The model under review builds one solid part; all positions refer to its coordinate system, in mm. Face numbers are marked on the shaded views. A direction names the side the tool comes from. Coordinates: 2 decimals unless noted, no trailing zeros. Order: outer loops, then holes, each group sorted by start corner. A loop starts at its lowest first (then second) coordinate and runs counter-clockwise, first axis right, second up. Notation, with made-up numbers: (87.5, -40) -> (125.5, -40) arc R16 ccw to (125.5, -10) -> close; hole circle Ø2 at (-2.75, -34.75). An arc over 180 degrees is marked (long way). Use one line per item in the form item = value.
from build123d import *

# Parameters (mm, degrees)
SKETCH_R           = 15
PAD_DEPTH          = 108
PAD_TAPER          = -10
SKETCH001_R        = 72.5
PAD001_DEPTH       = 14
POCKET_DEPTH       = 571.52662
PAD002_DEPTH       = 2.5
POLARPATTERN_COUNT = 6


with BuildPart() as part:
    # Sketch (on XY_Plane of Origin) → Pad (new body)
    with BuildSketch(Plane.XY):
        Circle(SKETCH_R)
    extrude(amount=-PAD_DEPTH, taper=PAD_TAPER)

    # Sketch001 (on Face3 of Pad) → Pad001 (join)
    with BuildSketch(Plane(origin=(0, 0, -108), x_dir=(1, 0, 0), z_dir=(0, 0, -1))):
        Circle(SKETCH001_R)
    extrude(amount=-PAD001_DEPTH)

    # Sketch002 (on XY_Plane of Origin) → Pocket (cut, through all)
    with BuildSketch(Plane.XY):
        with BuildLine():
            Line((-31.369354, -65.362173), (-22.5, -50))
            Line((-22.5, -50), (22.5, -50))
            Line((22.5, -50), (31.369354, -65.362173))
            ThreePointArc((-31.369354, -65.362173), (0, -72.5), (31.369354, -65.362173))
        make_face()
    pocket = extrude(amount=-POCKET_DEPTH, mode=Mode.SUBTRACT)

    # Mirrored: Pocket across XZ
    add(pocket.mirror(Plane.XZ), mode=Mode.SUBTRACT)

    # Sketch003 (on XZ_Plane of Origin) → Groove (revolve, cut)
    with BuildSketch(Plane.XZ):
        Polygon((9.922867, 0), (28.966181, -108), (0, -108), (0, 0), align=None)
    revolve(axis=Axis((0, 0, 0), (0, 0, 1)), mode=Mode.SUBTRACT)

    # Sketch004 (on XZ_Plane of Origin) → Pad002 (join, symmetric)
    with BuildSketch(Plane.XZ):
        Polygon((31.369354, -94), (45, -94), (18.959115, -22.453256), (13.881982, -22.453256), (26.497603, -94), align=None)
    pad002 = extrude(amount=PAD002_DEPTH, both=True)

    # PolarPattern: Pad002 ×6 about axis
    polarpattern_axis = Axis((0, 0, 0), (0, 0, 1))
    for i in range(1, POLARPATTERN_COUNT):
        add(pad002.rotate(polarpattern_axis, i * 360 / POLARPATTERN_COUNT))


solid = part.part
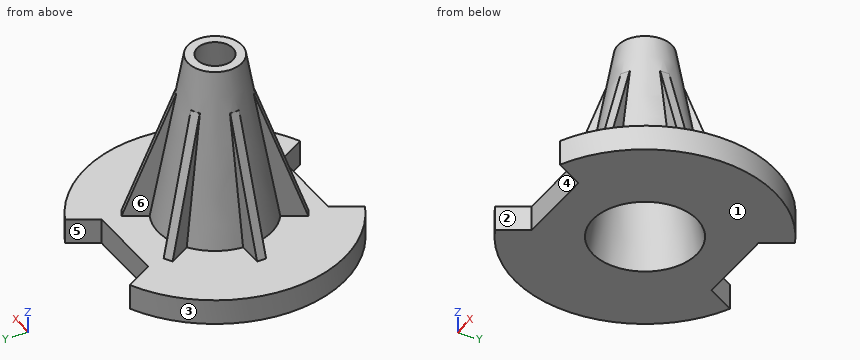
Item 1: Draft analysis for pull direction X (two halves, no side actions). For the marked faces 1, 2 and 3, state which applies: released by +X, released by -X, zero draft, split by the parting line, or undercut.
Results found:
face_1 = zero draft
face_2 = undercut
face_3 = released by -X
Item 2: Clearance check with flat-ended pins moving along their axes: pin 1 (10 mm diameter, centred on x = -44.5, z = -88.5, fed in from -Y); pin 2 (15.5 mm diameter, centred on x = -8, z = -99.5, fed in from -Y); pin 3 (12 mm diameter, centred on x = 26, z = -39.5, fed in from -Y). State where each tip first meets the part, or that it passes through.
Results found:
pin_1 = -2.5
pin_2 = -50
pin_3 = -9.32
Item 3: We need section D-D (y = 34). Write out the cut boundary in (x, z).
Results found:
outline = (-64.03, -108) -> (64.03, -108) -> (64.03, -94) -> (22.52, -94) -> (22.52, -82.19) -> (16.74, -74.26) -> (16.74, -94) -> (-16.74, -94) -> (-16.74, -74.26) -> (-22.52, -82.19) -> (-22.52, -94) -> (-64.03, -94) -> close
Item 4: Tool access review of the marked faces 4, 5 and 6: name each direction out of +Z, -Z, +X, -X, +Y, -Y from which nothing blocks a thin tool from reaching the whole face with its end or side.
Results found:
face_4 = +Z, -Z, -Y
face_5 = +Z, -Z, +Y
face_6 = +Z, +Y
Item 5: To check wall thickness, follow L1, parallel to Y at x = 19, z = -76; L2, parallel to Y at x = 20.5, z = -79; L3, parallel to X at y = -15, z = -97.5. State the ranges of each line that lie inside material, in increasing order. Write a range as from..to.
Results found:
L1 = -33.43..-27.91, -21.11..-13.53, 13.53..21.11, 27.91..33.43
L2 = -33.82..-30.51, -20.41..-12.19, 12.19..20.41, 30.51..33.82
L3 = -70.93..-22.59, 22.59..70.93
Item 6: We need section C-C (x = 0). Write out the cut boundary in (y, z).
Results found:
outline = (-50, -108) -> (-28.97, -108) -> (-9.92, 0) -> (-15, 0) -> (-31.57, -94) -> (-50, -94) -> close; (9.92, 0) -> (28.97, -108) -> (50, -108) -> (50, -94) -> (31.57, -94) -> (15, 0) -> close
Item 7: We need section B-B (y = -52.5). Write out the cut boundary in (x, z), plus the area to 3 significant figures.
Results found:
outline = (-50, -108) -> (-23.94, -108) -> (-23.94, -94) -> (-50, -94) -> close; (23.94, -108) -> (50, -108) -> (50, -94) -> (23.94, -94) -> close
area = 730 mm²
Item 8: We need section A-A (z = -35.5). Write out the cut boundary in (x, y), plus the area to 3 significant figures.
Results found:
outline = (-23.71, -2.5) -> (-21.11, -2.5) arc R21.26 ccw to (-12.72, -17.03) -> (-14.02, -19.28) -> (-9.69, -21.78) -> (-8.39, -19.53) arc R21.26 ccw to (8.39, -19.53) -> (9.69, -21.78) -> (14.02, -19.28) -> (12.72, -17.03) arc R21.26 ccw to (21.11, -2.5) -> (23.71, -2.5) -> (23.71, 2.5) -> (21.11, 2.5) arc R21.26 ccw to (12.72, 17.03) -> (14.02, 19.28) -> (9.69, 21.78) -> (8.39, 19.53) arc R21.26 ccw to (-8.39, 19.53) -> (-9.69, 21.78) -> (-14.02, 19.28) -> (-12.72, 17.03) arc R21.26 ccw to (-21.11, 2.5) -> (-23.71, 2.5) -> close; hole circle Ø32.36 at (0, 0)
area = 672 mm²
